Source: CAD feature listing. Evaluate the final solid. Frame: model axes, mm. A direction names the side the tool comes from. Give positions to 0.01 mm unless a question says otherwise; leave off trailing zeros. Order: outer loops, then holes, each group sorted by start corner. A loop starts at its lowest first (then second) coordinate and runs counter-clockwise, first axis right, second up.
from build123d import *

# Parameters (mm, degrees)
F0_R          = 63.5
F1_DEPTH      = 254
F1_TAPER      = -20
F1_DEPTH_BACK = 254
F1_TAPER_BACK = -20
F2_R          = 25.4
F3_SIZE       = 63.5
F4_T          = -12.7


# Not quite as in the source:
# - a shell that OpenCascade refuses in one call is made with other operations: the cavity is built on its own and cut out


with BuildPart() as f1:
    # F0 (on Front) → F1 (new body, two sides)
    with BuildSketch(Plane.XZ) as f1_sk:
        Circle(F0_R)
    extrude(amount=F1_DEPTH, taper=F1_TAPER)
    extrude(f1_sk.sketch, amount=-F1_DEPTH_BACK, taper=F1_TAPER_BACK)

    # F2
    f2_edges = [f1.edges().sort_by_distance(p)[0] for p in [
        (-155.94844, -254, 0),
    ]]
    fillet(f2_edges, radius=F2_R)

    # F3
    f3_edges = [f1.edges().sort_by_distance(p)[0] for p in [
        (-155.94844, 254, 0),
    ]]
    chamfer(f3_edges, length=F3_SIZE)

    # F4: a shell. OpenCascade refuses it in one call, so the cavity is built on its own and cut out:
    # the body offset inwards by the wall thickness, plus a prism from it out through each open face.
    f4_core = offset(f1.part, amount=F4_T, kind=Kind.INTERSECTION, mode=Mode.PRIVATE)
    f4_exits = [f4_core.faces().sort_by_distance(p)[0] for p in [
        (0, -241.3, 0),
    ]]
    add(f4_core, mode=Mode.SUBTRACT)
    extrude(f4_exits, amount=-F4_T, mode=Mode.SUBTRACT)


solid = f1.part
(1) Section C-C, the plane x = 0. Return loops of the section in (y, z).
(2) Section A-A, the plane z = 109.5. Count the separate pieces of the cut face and the enclosed holes in it, plus the area to 3 significant figures.
(3) Draft query along X for faces 3 (the flat face through (-1, 241.3, 1)), 4 (the conical face through (-74.974, 251.103, -57.488)), 5 (the flat face through (-1, 254, 1)). Return one class per face: +X half, -X half, draft (parallel to the pull), parting line (faces both ways), or undercut.
(4) Line query: line 1 along X through (y, z) = (-251, 0); line 2 along X through (y, z) = (-249.5, 0); line 3 along Y through (x, z) = (-80.5, -71). Output: solid intervals per line, ascending.
(5) Pin query (flat end, axial travel): pin 1 Ø2 at (x, y) = (109.5, -189.5) entering from -Z; pin 2 Ø5 at (x, y) = (-110.5, 183.5) entering from -Z; pin 3 Ø10 at (x, z) = (-98, -42) entering from +Y. Return the tip coordinate at first contact, or that it passes through.
(6) Access query for faces 1 (the cylindrical face through (-15.579, -247.561, -118.655)), 2 (the conical face through (74.13, 76.19, 23.34)). Directions: +Z, -Z, +X, -X, +Y, -Y. A direction counts if a zero-diameter tool reaches every point of the face in a straight line with its end or side. Return the directions, or none.
Checks:
1. outline: (-254, -119.67) arc R25.4 ccw to (-219.91, -143.54) - (0, -63.5) - (194.33, -134.23) - (254, -92.45) - (254, 92.45) - (194.33, 134.23) - (0, 63.5) - (-219.91, 143.54) arc R25.4 ccw to (-254, 119.67) - (-241.3, 119.67) arc R12.7 cw to (-224.26, 131.61) - (0, 49.98) - (192.46, 120.03) - (241.3, 85.84) - (241.3, -85.84) - (192.46, -120.03) - (0, -49.98) - (-224.26, -131.61) arc R12.7 cw to (-241.3, -119.67) - close
2. separate pieces: 2
2. enclosed holes: 1
2. area: 15,500 mm2
3. face 3: undercut
3. face 4: parting line
3. face 5: draft
4. line 1: x = -131.65 to -119.67, 119.67 to 131.65
4. line 2: x = -134.11 to -119.67, 119.67 to 134.11
4. line 3: y = -157.57 to -120.44, 120.44 to 157.57, 210.6 to 232.74
5. pin 1: stops at z = -76.14
5. pin 2: stops at z = -73.22
5. pin 3: stops at y = 240.9
6. face 1: -Y
6. face 2: none
